```python
from build123d import *

# Parameters (mm, degrees)
F0_R     = 25.4
F1_DEPTH = 6.35
F3_DEPTH = 12.7
F5_COUNT = 6
F6_R     = 6.47642
F7_DEPTH = 12.7
F8_R     = 16.375735
F9_DEPTH = 12.7


with BuildPart() as f1:
    # F0 (on Front) → F1 (new body, symmetric)
    with BuildSketch(Plane.XZ):
        Circle(F0_R)
    extrude(amount=F1_DEPTH, both=True)

    # F2 (on face) → F3 (join)
    with BuildSketch(Plane.XZ.offset(6.35)):
        Polygon((-0.289307, 0), (0, 0), (-24.534516, 6.574004), (-24.534516, 6.47642), (-24.459638, 6.47642), align=None)
        Polygon((-24.534516, -6.574004), (0, 0), (-0.289307, 0), (-24.459638, -6.47642), (-24.534516, -6.47642), align=None)
        Polygon((-24.534516, 0), (-24.534516, 6.47642), (-34.619638, 6.47642), (-34.619638, -6.47642), (-24.534516, -6.47642), align=None)
    extrude(amount=-F3_DEPTH)

    # F5: F1 ×6 about axis
    f5_axis = Axis((0, -23.88444, 0), (0, -1, 0))


with BuildPart() as f1_1:
    add(f1.part)
    for i in range(1, F5_COUNT):
        add(f1.part.rotate(f5_axis, i * 360 / F5_COUNT))

    # F6 (on face) → F7 (cut)
    with BuildSketch(Plane.XZ.offset(6.35)):
        Circle(F6_R)
    extrude(amount=F7_DEPTH, mode=Mode.SUBTRACT)

    # F8 (on face) → F9 (cut)
    with BuildSketch(Plane(origin=(0, 6.35, 0), x_dir=(-1, 0, 0), z_dir=(0, 1, 0))):
        Circle(F8_R)
    extrude(amount=-F9_DEPTH, mode=Mode.SUBTRACT)


solid = f1_1.part
```
The listing builds one solid part. Answer for the finished solid, in the listing's coordinates (mm). A direction names the side the tool comes from. Coordinates: 2 decimals unless noted, no trailing zeros. Write each loop counter-clockwise with the first axis right and the second up, starting at its lowest first coordinate (ties: lowest second). Pieces come first, ordered by that corner, then holes. Notation, with made-up numbers: (52, 25) -> (84, 25) arc R15 ccw to (84, 41) -> close; hole circle Ø8 at (-6.75, 77.25). An arc over 180 degrees is marked (long way). Write each question's results on one line, items separated by ' | '. Start each with the question number.
1) A cutting plane is placed at D-D (x = -29). Determine the outline of the cut face in (y, z), then the cut area to 3 significant figures.
2) A cutting plane is placed at A-A (z = 0). Determine the outline of the cut face in (x, y).
3) A cutting plane is placed at B-B (y = 0.5). Determine the outline of the cut face in (x, z), then the cut area to 3 significant figures.
4) Straight lines are drawn through the part: probe 1 along X at (y, z) = (5, 0.5); probe 2 along Z at (x, y) = (-18.5, 4); probe 3 along Z at (x, y) = (-21, 0.25). For each, find the intervals that lie inside material, in ascending order.
5) Flat-ended cylindrical pins translate along their axes: pin 1 Ø4 at (x, y) = (-27.5, -3.5) entering from -Z; pin 2 Ø5 at (x, y) = (31.5, 1.5) entering from +Z; pin 3 Ø3 at (x, y) = (-25, 2) entering from +Z. Find the tip coordinate at first contact, or state that the pin passes through.
6) A tool of negligible diameter and unlimited length cuts with its end or side. For faces 5 (the flat face through (20.44, -0.09, -22.45)), 6 (the cylindrical face through (-22.044, -0.089, -12.618)), 7 (the flat face through (30, 0, -6.476)), 8 (the flat face through (-9.15, -0.09, 28.8)), 9 (the flat face through (17.388, -0.089, 29.936)), from which of +Z, -Z, +X, -X, +Y, -Y can it reach the whole face along a straight path? Write none if from no direction.
7) For a pull along X with two mould halves and no side action, classify faces 1 (the flat face through (9.22, -0.09, 28.92)), 2 (the flat face through (9.15, -0.09, -28.8)), 3 (the flat face through (-30, 0, 6.476)), 4 (the flat face through (-17.231, -0.089, 30.027)) as +X half, -X half, draft (parallel to the pull), parting line (faces both ways), or undercut.
8) A cutting plane is placed at C-C (x = 0). Determine the outline of the cut face in (y, z).
Values follow:
1) outline: (-6.35, -6.48) -> (6.35, -6.48) -> (6.35, 6.48) -> (-6.35, 6.48) -> close | area: 165 mm²
2) outline: (-34.62, -6.35) -> (-16.38, -6.35) -> (-16.38, 6.35) -> (-34.62, 6.35) -> close; (16.38, -6.35) -> (34.62, -6.35) -> (34.62, 6.35) -> (16.38, 6.35) -> close
3) outline: (-34.62, -6.48) -> (-24.56, -6.48) arc R25.4 ccw to (-17.89, -18.03) -> (-22.92, -26.74) -> (-11.7, -33.22) -> (-6.67, -24.51) arc R25.4 ccw to (6.67, -24.51) -> (11.7, -33.22) -> (22.92, -26.74) -> (17.89, -18.03) arc R25.4 ccw to (24.56, -6.48) -> (34.62, -6.48) -> (34.62, 6.48) -> (24.56, 6.48) arc R25.4 ccw to (17.89, 18.03) -> (22.92, 26.74) -> (11.7, 33.22) -> (6.67, 24.51) arc R25.4 ccw to (-6.67, 24.51) -> (-11.7, 33.22) -> (-22.92, 26.74) -> (-17.89, 18.03) arc R25.4 ccw to (-24.56, 6.48) -> (-34.62, 6.48) -> close; hole circle Ø32.75 at (0, 0) | area: 1,920 mm²
4) probe 1: -34.62 to -16.37, 16.37 to 34.62 | probe 2: -29.29 to -19.09, -17.4 to 17.4, 19.09 to 29.29 | probe 3: -27.85 to -23.42, -14.29 to 14.29, 23.42 to 27.85
5) pin 1: z = -6.48 | pin 2: z = 6.48 | pin 3: z = 9.64
6) face 5: +X, +Y, -Y | face 6: -X, +Y, -Y | face 7: -Z, +X, +Y, -Y | face 8: +Z, +Y, -Y | face 9: +Z, +X, +Y, -Y
7) face 1: undercut | face 2: undercut | face 3: draft | face 4: -X half
8) outline: (-6.35, -25.4) -> (6.35, -25.4) -> (6.35, -16.38) -> (-6.35, -16.38) -> close; (-6.35, 16.38) -> (6.35, 16.38) -> (6.35, 25.4) -> (-6.35, 25.4) -> close
